Geometry: final body of the model. Coordinates: model frame, mm. A direction names the side the tool comes from. Give positions to 0.01 mm unless a question says otherwise; leave off trailing zeros.
```python
from build123d import *

# Parameters (mm, degrees)
BOSS_EXTRUDE1_DEPTH = 100


with BuildPart() as part:
    # Sketch4 → Boss-Extrude1 (new body, symmetric)
    with BuildSketch(Plane.XY):
        with BuildLine():
            Line((4.8, -20), (17.2, -20))
            ThreePointArc((17.2, -20), (19.179898987, -19.179898987), (20, -17.2))
            Line((20, -17.2), (20, -4.8))
            ThreePointArc((20, -4.8), (19.765685425, -4.234314575), (19.2, -4))
            Line((19.2, -4), (16.190663761, -4))
            ThreePointArc((16.190663761, -4), (15.624978336, -4.234314575), (15.390663761, -4.8))
            Line((15.390663761, -4.8), (15.390663761, -10.2))
            ThreePointArc((15.390663761, -10.2), (14.896810507, -10.939103626), (14.024978336, -10.765685425))
            Line((14.024978336, -10.765685425), (9.40588745, -6.146594539))
            ThreePointArc((9.40588745, -6.146594539), (8.365378244, -4.589362465), (8, -2.752481989))
            Line((8, -2.752481989), (8, 0))
            Line((8, 0), (3.5, 0))
            ThreePointArc((3.5, 0), (2.474873734, -2.474873734), (0, -3.5))
            Line((0, -3.5), (0, -8))
            Line((0, -8), (2.752481989, -8))
            ThreePointArc((2.752481989, -8), (4.589362465, -8.365378244), (6.146594539, -9.40588745))
            Line((6.146594539, -9.40588745), (10.765685425, -14.024978336))
            ThreePointArc((10.765685425, -14.024978336), (10.939103626, -14.896810507), (10.2, -15.390663761))
            Line((10.2, -15.390663761), (4.8, -15.390663761))
            ThreePointArc((4.8, -15.390663761), (4.234314575, -15.624978336), (4, -16.190663761))
            Line((4, -16.190663761), (4, -19.2))
            ThreePointArc((4, -19.2), (4.234314575, -19.765685425), (4.8, -20))
        make_face()
    extrude(amount=BOSS_EXTRUDE1_DEPTH, both=True)

    # Mirror1: part across plane


with BuildPart() as part_1:
    add(part.part)
    add(part.part.mirror(Plane(origin=(0, 0, 0), x_dir=(0, 0, 1), z_dir=(1, 0, 0))))

    # Mirror2: part across plane


with BuildPart() as part_2:
    add(part_1.part)
    add(part_1.part.mirror(Plane.ZX))


solid = part_2.part
```
Item 1: Reachability of faces 1 (the face through (-8, -15.391, 1)), 2 (the face through (8, 0, 1)), 3 (the face through (20, 11, 1)) from +Z, -Z, +X, -X, +Y, -Y: full face, straight path, thin tool, end or side. Return the list, or none.
Found:
face 1: +Z, -Z
face 2: +Z, -Z, +X
face 3: +Z, -Z, +X, +Y, -Y
Item 2: Pin query (flat end, axial travel): pin 1 Ø3 at (y, z) = (-1, -20.5) entering from -X; pin 2 Ø6 at (x, z) = (0, -1.5) entering from +Y; pin 3 Ø0.9 at (x, z) = (-18, 6.5) entering from -Y. Return the tip coordinate at first contact, or that it passes through.
Found:
pin 1: stops at x = -8
pin 2: stops at y = 8.01
pin 3: stops at y = -19.98
Item 3: Line query: L1, parallel to Y at x = 16, z = 31; L2, parallel to Y at x = -9.5, z = -90. Output: solid intervals per line, ascending.
Found:
L1: y = -20 to -4.02, 4.02 to 20
L2: y = -20 to -15.39, -12.76 to -6.24, 6.24 to 12.76, 15.39 to 20
Item 4: Pull-direction query (Y, two-part tool) for faces 4 (the face through (11, 20, 1)), 5 (the face through (15.391, -7, 1)), 6 (the face through (8.42, -11.68, 1.4)), 7 (the face through (-20, -11, 1)); classes: +Y half, -Y half, draft (parallel to the pull), parting line (faces both ways), or undercut.
Found:
face 4: +Y half
face 5: undercut
face 6: undercut
face 7: draft
